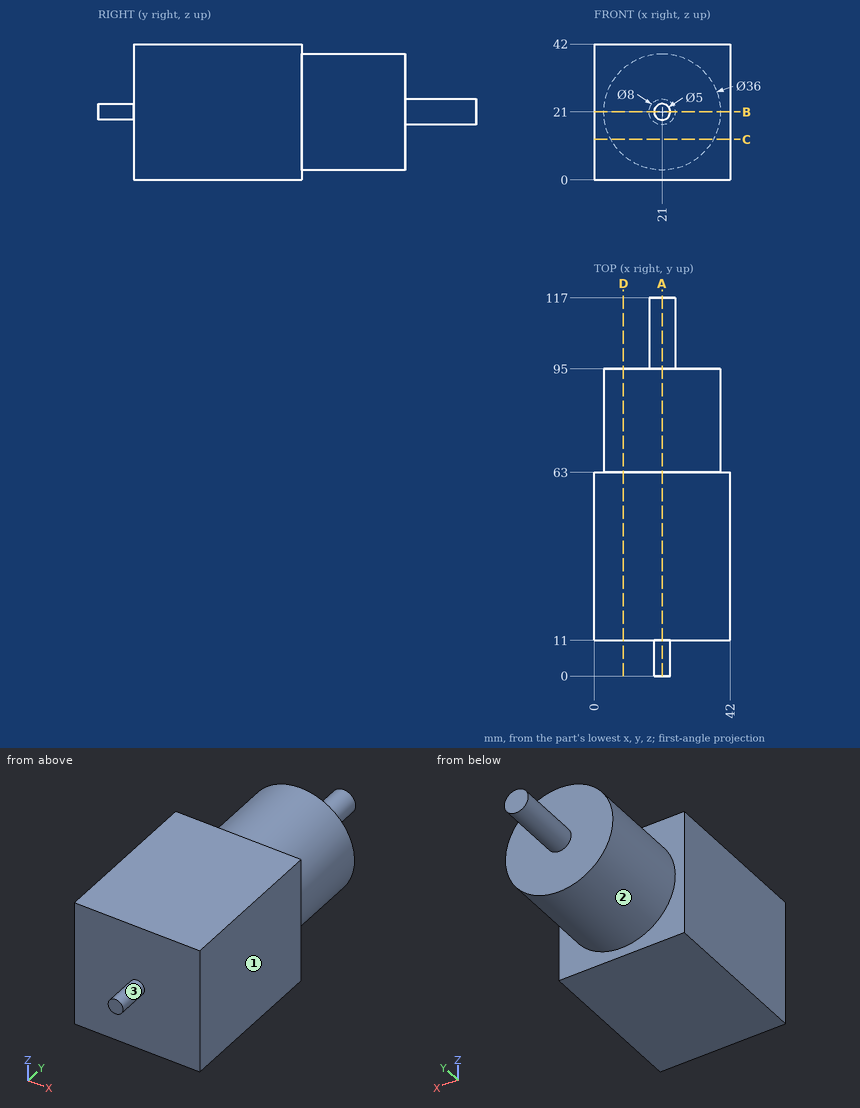
Answer from the drawing. Dimensions are ordinates in mm from the lowest x, y and z of the part. A direction names the side the tool comes from. Give positions to 0.01 mm unless a question says otherwise; leave off trailing zeros. Loops run counter-clockwise (first coordinate to the right, second up) from the corner with the lowest first, then second, coordinate; pieces in that order, holes last. Notation, with made-up numbers: (37.5, -6) - (66.5, -6) arc R26 ccw to (66.5, 32) - close; hole circle Ø7 at (53, 45.25). An arc over 180 degrees is marked (long way). Write each question's results on one line, items separated by ' | '.
1. Consider probe 1 along Y at (x, z) = (16, 37); probe 2 along Y at (x, z) = (2.5, 11.5); probe 3 along Z at (x, y) = (15, 67.5). Determine where each line is inside the solid, lowest interval first. Write a range as from..to.
Resolved:
probe 1: y = 11..95 | probe 2: y = 11..63 | probe 3: z = 4.03..37.97
2. Find section A-A, the plane x = 21. Write down the section's boundary in (y, z), then the cut area to 3 significant figures.
Resolved:
outline: (0, 18.5) - (11, 18.5) - (11, 0) - (63, 0) - (63, 3) - (95, 3) - (95, 17) - (117, 17) - (117, 25) - (95, 25) - (95, 39) - (63, 39) - (63, 42) - (11, 42) - (11, 23.5) - (0, 23.5) - close | area: 3,570 mm^2
3. Find section B-B, the plane z = 21. Write down the section's boundary in (x, y).
Resolved:
outline: (0, 11) - (18.5, 11) - (18.5, 0) - (23.5, 0) - (23.5, 11) - (42, 11) - (42, 63) - (39, 63) - (39, 95) - (25, 95) - (25, 117) - (17, 117) - (17, 95) - (3, 95) - (3, 63) - (0, 63) - close
4. Find section C-C, the plane z = 12.5. Write down the section's boundary in (x, y), then the cut area to 3 significant figures.
Resolved:
outline: (0, 11) - (42, 11) - (42, 63) - (36.87, 63) - (36.87, 95) - (5.13, 95) - (5.13, 63) - (0, 63) - close | area: 3,200 mm^2
5. Flat-ended cylindrical pins translate along their axes: P1, Ø3, axis at x = 22, z = 6, coming from the +Y side; P2, Ø6, axis at y = 81, z = 10.5, coming from the -X side; P3, Ø10, axis at x = 37, z = 26.5, coming from the -Y side. Find the tip coordinate at first contact, or state that the pin passes through.
Resolved:
P1: stops at y = 95 | P2: stops at x = 4.64 | P3: stops at y = 11
6. Find section D-D, the plane x = 9. Write down the section's boundary in (y, z), then the cut area to 3 significant figures.
Resolved:
outline: (11, 0) - (63, 0) - (63, 7.58) - (95, 7.58) - (95, 34.42) - (63, 34.42) - (63, 42) - (11, 42) - close | area: 3,040 mm^2
7. Which of the six approach directions +Z, -Z, +X, -X, +Y, -Y give full straight-line access (tool end or side, diameter ignored) to the marked faces 1, 2 and 3?
Resolved:
face 1: +Z, -Z, +X, +Y, -Y | face 2: +Y | face 3: -Y
